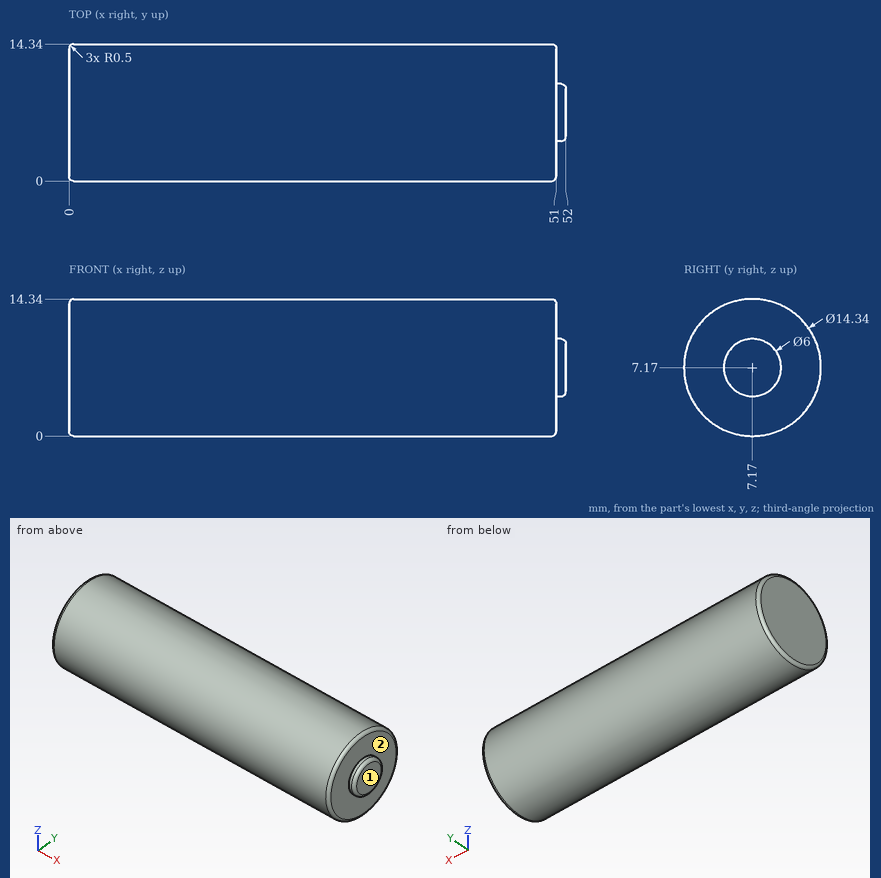
The figure shows three views and two pictorial views of one solid part (mm, origin at its lowest corner). Answer the questions. A direction names the side the tool comes from. Round coordinates to 2 decimals unless told otherwise and drop trailing zeros. Answer as a JSON object with one key per item and string values. Group by question number.
Q1. Each of these flat-tipped pins is pushed along its axis until it touches: pin 1 Ø4 at (x, y) = (45.5, 1.5) entering from -Z; pin 2 Ø2 at (x, y) = (12, 5.5) entering from +Z; pin 3 Ø5 at (x, y) = (20, 4) entering from -Z. Where does it stop, or does it pass through?
Q2. Which of the six approach directions +Z, -Z, +X, -X, +Y, -Y give full straight-line access (tool end or side, diameter ignored) to the marked faces 1 and 2?
Q3. Straight lines are drawn through the part: line 1 along X through (y, z) = (4, 4.5); line 2 along Y through (x, z) = (27, 12.5); line 3 along Z through (x, y) = (33, 4.25). For each, find the intervals that lie inside material, in ascending order.
Check values:
{
 "1": {"pin 1": "z = 1.01", "pin 2": "z = 14.31", "pin 3": "z = 0.03"},
 "2": {"face 1": "+Z, -Z, +X, +Y, -Y", "face 2": "+X"},
 "3": {"line 1": "0 to 51", "line 2": "2.37 to 11.97", "line 3": "0.62 to 13.72"}
}
